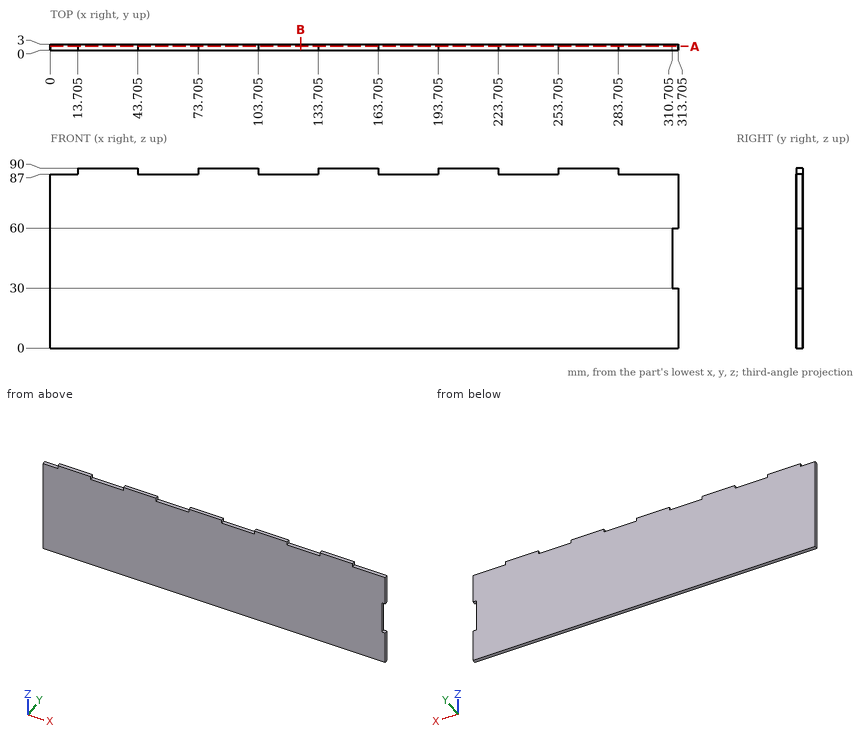
Can you work these out from the drawing? Everything is in mm from the part's minimum corner. Coordinates: 2 decimals unless noted, no trailing zeros. Write each loop counter-clockwise with the first axis right and the second up, starting at its lowest first coordinate (ties: lowest second). Pieces come first, ordered by that corner, then holes. Notation, with made-up numbers: (19, -11) - (69, -11) arc R19 cw to (69, -5) - close; hole circle Ø3 at (82, -18.75). An arc over 180 degrees is marked (long way). One line per item, written item: value.
1) I need wall thicknesses on line 1 along X through (y, z) = (0.2, 38.5) (3 decimals); line 2 along Z through (x, y) = (292.5, 0.3). Which ranges of each line are inside material? Lowest first, please.
Model answer:
line 1: x = 0 to 310.705
line 2: z = 0 to 87
2) Suppose I cut it at A-A on y = 1.85. Write out the boundary of the cut face in (x, z) (3 decimals).
Model answer:
outline: (0, 0) - (313.705, 0) - (313.705, 30) - (310.705, 30) - (310.705, 60) - (313.705, 60) - (313.705, 87) - (283.705, 87) - (283.705, 90) - (253.705, 90) - (253.705, 87) - (223.705, 87) - (223.705, 90) - (193.705, 90) - (193.705, 87) - (163.705, 87) - (163.705, 90) - (133.705, 90) - (133.705, 87) - (103.705, 87) - (103.705, 90) - (73.705, 90) - (73.705, 87) - (43.705, 87) - (43.705, 90) - (13.705, 90) - (13.705, 87) - (0, 87) - close
3) I'm going to push flat-ended pins straight in: P1, Ø1.5, axis at y = 1.5, z = 89, coming from the +X side (3 decimals); P2, Ø0.9, axis at x = 126, y = 2, coming from the +Z side; P3, Ø0.9, axis at y = 1.5, z = 89, coming from the -X side (3 decimals). Where does each tip first touch, or does it pass through?
Model answer:
P1: stops at x = 283.705
P2: stops at z = 87
P3: stops at x = 13.705
4) Suppose I cut it at B-B on x = 125. Write out the boundary of the cut face in (y, z), and give its area (3 significant figures).
Model answer:
outline: (0, 0) - (3, 0) - (3, 87) - (0, 87) - close
area: 261 mm²
